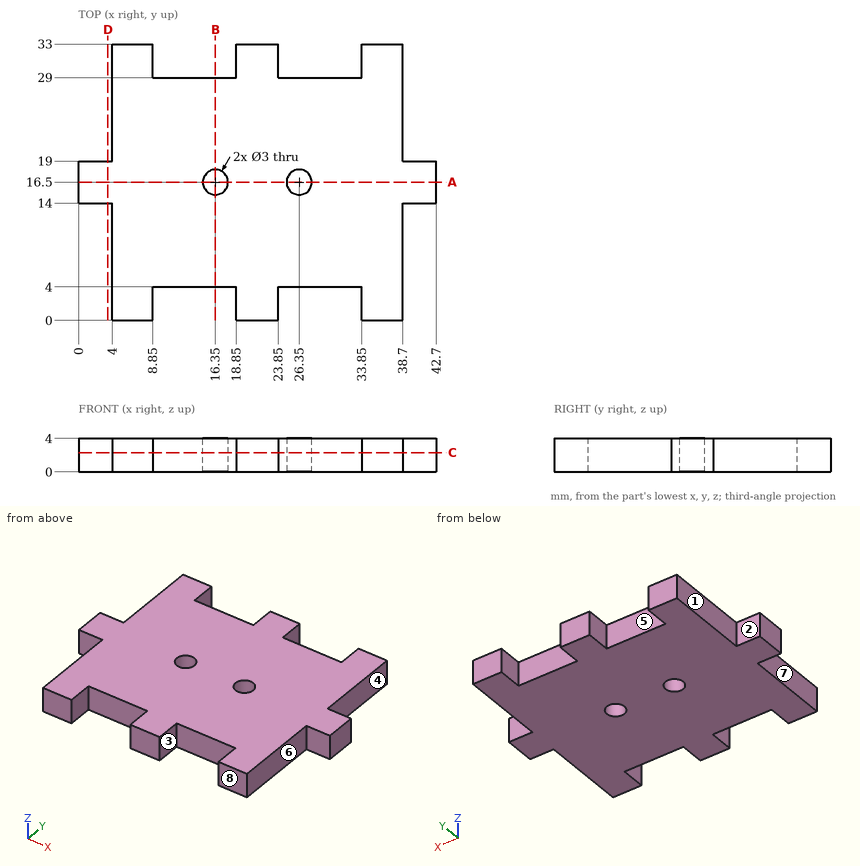
The figure shows three views and two pictorial views of one solid part (mm, origin at its lowest corner). Answer the questions. A direction names the side the tool comes from. Round coordinates to 2 decimals unless told otherwise and drop trailing zeros. Write each loop counter-clockwise with the first axis right and the second up, starting at its lowest first coordinate (ties: lowest second). Pieces come first, ordered by that corner, then holes. Notation, with made-up numbers: M 10.5,-4.75 L 68.5,-4.75 A31 cw 68.5,31.25 Z; hole C 15,20.5 d2. An arc over 180 degrees is marked long. Use a Markdown table: item, result.
1) The part is cut by section D-D (x = 3.5). Write down the section's boundary in (y, z), plus the area to 3 significant figures.
Answers follow:
| item | result |
|---|---|
| outline | M 14,0 L 19,0 L 19,4 L 14,4 Z |
| area | 20.0 mm2 |
2) A tool of negligible diameter and unlimited length cuts with its end or side. For the marked faces 4, 5, 6, 7 and 8, from which of +Z, -Z, +X, -X, +Y, -Y can it reach the whole face along a straight path? Write none if from no direction.
Answers follow:
| item | result |
|---|---|
| face 4 | +Z, -Z, +X, +Y |
| face 5 | +Z, -Z, +Y |
| face 6 | +Z, -Z, +X, -Y |
| face 7 | +Z, -Z, -X, -Y |
| face 8 | +Z, -Z, +X, -X, -Y |
3) Straight lines are drawn through the part: line 1 along X through (y, z) = (30, 0.7); line 2 along Y through (x, z) = (16.35, 2.95); line 3 along Y through (x, z) = (24, 2.3). For each, find the intervals that lie inside material, in ascending order. Write a range as [from, to].
Answers follow:
| item | result |
|---|---|
| line 1 | x = [4, 8.85], [18.85, 23.85], [33.85, 38.7] |
| line 2 | y = [4, 15], [18, 29] |
| line 3 | y = [4, 29] |
4) The part is cut by section B-B (x = 16.35). Write down the section's boundary in (y, z), plus the area to 3 significant figures.
Answers follow:
| item | result |
|---|---|
| outline | M 4,0 L 15,0 L 15,4 L 4,4 Z; M 18,0 L 29,0 L 29,4 L 18,4 Z |
| area | 88.0 mm2 |
5) For a pull along X with two mould halves and no side action, classify the marked faces 1, 2 and 3 as pulls with the +X half, pulls with the -X half, needs draft (parallel to the pull), parting line crosses it, or undercut.
Answers follow:
| item | result |
|---|---|
| face 1 | pulls with the -X half |
| face 2 | needs draft |
| face 3 | undercut |
6) The part is cut by section A-A (y = 16.5). Write down the section's boundary in (x, z), plus the area to 3 significant figures.
Answers follow:
| item | result |
|---|---|
| outline | M 0,0 L 14.85,0 L 14.85,4 L 0,4 Z; M 17.85,0 L 24.85,0 L 24.85,4 L 17.85,4 Z; M 27.85,0 L 42.7,0 L 42.7,4 L 27.85,4 Z |
| area | 147 mm2 |
7) The part is cut by section C-C (z = 2.3). Give the number of separate pieces and of enclosed holes in the cut face, plus the area to 3 significant figures.
Answers follow:
| item | result |
|---|---|
| separate pieces | 1 |
| enclosed holes | 2 |
| area | 1,010 mm2 |
8) Flat-ended cylindrical pins translate along their axes: pin 1 (2 mm diameter, centred on y = 27.5, z = 1, fed in from -X); pin 2 (1.2 mm diameter, centred on y = 26, z = 1, fed in from +X); pin 3 (2 mm diameter, centred on x = 16, z = 1.5, fed in from +Y); pin 4 (1.8 mm diameter, centred on x = 16.35, y = 16.5, fed in from +Z). Find the tip coordinate at first contact, or state that the pin passes through.
Answers follow:
| item | result |
|---|---|
| pin 1 | stops at x = 4 |
| pin 2 | stops at x = 38.7 |
| pin 3 | stops at y = 29 |
| pin 4 | passes through |
